```python
from build123d import *

# Parameters (mm, degrees)
SKETCH1_R               = 4.826
BOSS_EXTRUDE1_DEPTH     = 12.7
SKETCH2_R               = 1.8415
CUT_EXTRUDE1_DEPTH      = 20.165748301
CUT_EXTRUDE1_DEPTH_BACK = 7.35


with BuildPart() as part:
    # Sketch1 → Boss-Extrude1 (new body)
    with BuildSketch(Plane.XY):
        with BuildLine():
            Line((0, 0), (38.1, 0))
            Line((38.1, 0), (38.1, 6.35))
            Line((38.1, 6.35), (29.010834454, 6.35))
            ThreePointArc((29.010834454, 6.35), (24.972383208, 8.802433287), (25.286109599, 13.516783004))
            ThreePointArc((25.286109599, 13.516783004), (19.05, 25.515748301), (12.813890401, 13.516783004))
            ThreePointArc((12.813890401, 13.516783004), (13.127616792, 8.802433287), (9.089165546, 6.35))
            Line((9.089165546, 6.35), (0, 6.35))
            Line((0, 6.35), (0, 0))
        make_face()
        with Locations((19.05, 17.895748301)):
            Circle(SKETCH1_R, mode=Mode.SUBTRACT)
    extrude(amount=BOSS_EXTRUDE1_DEPTH)

    # Sketch2 → Cut-Extrude1 (cut, two sides)
    with BuildSketch(Plane(origin=(0, 6.35, 0), x_dir=(1, 0, 0), z_dir=(0, 1, 0))) as cut_extrude1_sk:
        with Locations((6.35, -6.35)):
            Circle(SKETCH2_R)
        with Locations((31.75, -6.35)):
            Circle(SKETCH2_R)
    extrude(amount=CUT_EXTRUDE1_DEPTH, mode=Mode.SUBTRACT)
    extrude(cut_extrude1_sk.sketch, amount=-CUT_EXTRUDE1_DEPTH_BACK, mode=Mode.SUBTRACT)


solid = part.part
```
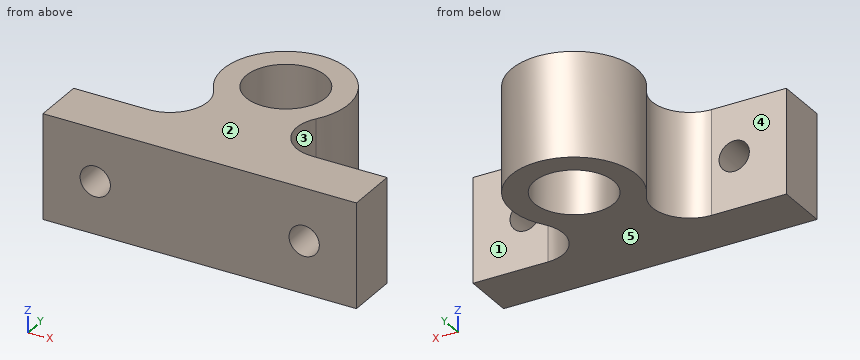
Geometry check sheet. Reference: the model listing, model coordinates, mm. Face numbers are marked on the shaded views. A direction names the side the tool comes from. Round coordinates to 2 decimals unless told otherwise and drop trailing zeros. Write each loop counter-clockwise with the first axis right and the second up, starting at its lowest first coordinate (ties: lowest second). Pieces come first, ordered by that corner, then holes. Notation, with made-up numbers: (36.5, 84.5) - (48.5, 84.5) arc R24 cw to (48.5, 109.5) - close; hole circle Ø11 at (-6.5, 47.5). An arc over 180 degrees is marked (long way). Write each question's results on one line, items separated by ' | '.
(1) Sectioned sample at B-B, the plane x = 31.75. Enter the section's corners in (y, z).
Computed:
outline: (0, 0) - (6.35, 0) - (6.35, 4.51) - (0, 4.51) - close; (0, 8.19) - (6.35, 8.19) - (6.35, 12.7) - (0, 12.7) - close
(2) Sectioned sample at C-C, the plane y = 19. Enter the section's corners in (x, z).
Computed:
outline: (11.51, 0) - (14.35, 0) - (14.35, 12.7) - (11.51, 12.7) - close; (23.75, 0) - (26.59, 0) - (26.59, 12.7) - (23.75, 12.7) - close
(3) Draft check along Y on the marked faces 3, 4 and 5. Enter one of: pulls with the +Y half, pulls with the -Y half, needs draft (parallel to the pull), parting line crosses it, or undercut.
Computed:
face 3: undercut | face 4: pulls with the +Y half | face 5: needs draft
(4) Sectioned sample at A-A, the plane z = 5.5. Enter the section's corners in (x, y), plus the area to 3 significant figures.
Computed:
outline: (0, 0) - (4.72, 0) - (4.72, 6.35) - (0, 6.35) - close; (7.98, 0) - (30.12, 0) - (30.12, 6.35) - (29.01, 6.35) arc R4.55 cw to (25.29, 13.52) arc R7.62 ccw (long way) to (12.81, 13.52) arc R4.55 cw to (9.09, 6.35) - (7.98, 6.35) - close; (33.38, 0) - (38.1, 0) - (38.1, 6.35) - (33.38, 6.35) - close; hole circle Ø9.65 at (19.05, 17.9) | area: 369 mm^2
(5) Depth check by flat-ended pin: pin 1 Ø1.5 at (x, y) = (22.5, 5.5) entering from -Z; pin 2 Ø1 at (x, y) = (11, 10) entering from -Z; pin 3 Ø7.5 at (x, z) = (31.5, 9) entering from +Y; pin 4 Ø4.5 at (x, z) = (5.5, 3.5) entering from +Y. Enter the tip coordinate at first touch or a pass-through.
Computed:
pin 1: stops at z = 0 | pin 2: passes through | pin 3: stops at y = 6.53 | pin 4: stops at y = 6.35
(6) Sectioned sample at D-D, the plane z = 10.25. Enter the section's corners in (x, y).
Computed:
outline: (0, 0) - (38.1, 0) - (38.1, 6.35) - (29.01, 6.35) arc R4.55 cw to (25.29, 13.52) arc R7.62 ccw (long way) to (12.81, 13.52) arc R4.55 cw to (9.09, 6.35) - (0, 6.35) - close; hole circle Ø9.65 at (19.05, 17.9)
(7) Set-up check for the marked faces 1 and 2: record each of +Z, -Z, +X, -X, +Y, -Y from which the full face is reachable in a straight line by a thin tool's end or side.
Computed:
face 1: +Z, -Z, +X, +Y | face 2: +Z, +X, -X, +Y, -Y
(8) Thickness scan on probe 1 along X at (y, z) = (3.5, 6.35); probe 2 along X at (y, z) = (3.75, 5.75); probe 3 along Y at (x, z) = (19.05, 2.5). Record the ranges inside material, lowest first. Write a range as from..to.
Computed:
probe 1: x = 0..4.51, 8.19..29.91, 33.59..38.1 | probe 2: x = 0..4.61, 8.09..30.01, 33.49..38.1 | probe 3: y = 0..13.07, 22.72..25.52
